Could you check a few things on this model? Use its own coordinates, in mm. A direction names the side the tool comes from. Round coordinates to 2 decimals unless told otherwise and drop trailing zeros. Loops run counter-clockwise (first coordinate to the right, second up) from the corner with the lowest first, then second, coordinate; pieces in that order, holes last. Notation, with made-up numbers: M -36,83.25 L -17,83.25 A9 cw -17,99.25 Z; hole C 77.5,-23.5 d11. An arc over 180 degrees is marked long. Answer in a Markdown table with one row per item.
```python
from build123d import *

# Parameters (mm, degrees)
SKETCH1_W           = 50
SKETCH1_H           = 170
BOSS_EXTRUDE1_DEPTH = 55
SKETCH2_W           = 34
SKETCH2_H           = 27
CUT_EXTRUDE1_DEPTH  = 181.416185527
SKETCH3_W           = 10
SKETCH3_H           = 24
SKETCH3_R           = 4.25
SKETCH3_R_2         = 1
CUT_EXTRUDE2_DEPTH  = 186.539753153
SKETCH4_W           = 2
SKETCH4_H           = 24
CUT_EXTRUDE3_DEPTH  = 178.623196683
SKETCH5_W           = 6.25
SKETCH5_H           = 11.25
CUT_EXTRUDE4_DEPTH  = 186.539753153
SKETCH6_W           = 38
SKETCH6_H           = 10
CUT_EXTRUDE5_DEPTH  = 181.416185527
SKETCH8_W           = 13.25
SKETCH8_H           = 2.25
CUT_EXTRUDE7_DEPTH  = 186.539753153
SKETCH9_W           = 34
SKETCH9_H           = 35.25
CUT_EXTRUDE8_DEPTH  = 179.297679458
SKETCH11_W          = 13.25
SKETCH11_H          = 20.25
CUT_EXTRUDE9_DEPTH  = 184.480414486
SKETCH12_W          = 28.5
SKETCH12_H          = 15
BOSS_EXTRUDE2_DEPTH = 8
SKETCH14_W          = 34
SKETCH14_H          = 15
SKETCH14_H_2        = 10.25
BOSS_EXTRUDE3_DEPTH = 13.25
SKETCH16_R          = 4.5
SKETCH16_R_2        = 2.5
CUT_EXTRUDE13_DEPTH = 8
SKETCH17_R          = 4.5
SKETCH17_W          = 55
SKETCH17_H          = 10.25
CUT_EXTRUDE15_DEPTH = 175.384811552
SKETCH18_W          = 71.25
SKETCH18_H          = 27.5
SKETCH18_W_2        = 13.75
SKETCH18_W_3        = 16.25
BOSS_EXTRUDE4_DEPTH = 50
SKETCH19_W          = 38
SKETCH19_H          = 7
CUT_EXTRUDE16_DEPTH = 152.25227271
SKETCH20_W          = 57.5
SKETCH20_H          = 27.5
CUT_EXTRUDE17_DEPTH = 102.137591923
CUT_EXTRUDE18_DEPTH = 100.39221549
SKETCH22_W          = 82.5
SKETCH22_H          = 2.5
BOSS_EXTRUDE5_DEPTH = 50
SKETCH24_W          = 22
SKETCH24_H          = 17
CUT_EXTRUDE19_DEPTH = 101.710289941
SKETCH25_W          = 38
SKETCH25_H          = 38.136363636
CUT_EXTRUDE20_DEPTH = 10


with BuildPart() as part:
    # Sketch1 → Boss-Extrude1 (new body)
    with BuildSketch(Plane.XY):
        with Locations((0, -85)):
            Rectangle(SKETCH1_W, SKETCH1_H)
    extrude(amount=-BOSS_EXTRUDE1_DEPTH)

    # Sketch2 → Cut-Extrude1 (cut, through all)
    with BuildSketch(Plane.XY):
        with Locations((0, -13.5)):
            Rectangle(SKETCH2_W, SKETCH2_H)
    extrude(amount=-CUT_EXTRUDE1_DEPTH, mode=Mode.SUBTRACT)

    # Sketch3 → Cut-Extrude2 (cut, through all)
    with BuildSketch(Plane(origin=(25, 0, 0), x_dir=(0, 0, -1), z_dir=(1, 0, 0))):
        with Locations((50, -12)):
            Rectangle(SKETCH3_W, SKETCH3_H)
        with Locations((5, -12)):
            Rectangle(SKETCH3_W, SKETCH3_H)
        with Locations(Location((27.5, -12.75, 0), (0, 0, 90))):
            Circle(SKETCH3_R)
        with Locations(Location((35.5, -12.75, 0), (0, 0, 90))):
            Circle(SKETCH3_R_2)
        with Locations(Location((27.5, -4.75, 0), (0, 0, 90))):
            Circle(SKETCH3_R_2)
        with Locations(Location((27.5, -20.75, 0), (0, 0, 90))):
            Circle(SKETCH3_R_2)
        with Locations(Location((19.5, -12.75, 0), (0, 0, 90))):
            Circle(SKETCH3_R_2)
    extrude(amount=-CUT_EXTRUDE2_DEPTH, mode=Mode.SUBTRACT)

    # Sketch4 → Cut-Extrude3 (cut, through all)
    with BuildSketch(Plane.XY.offset(-10)):
        with Locations((-18, -12)):
            Rectangle(SKETCH4_W, SKETCH4_H)
        with Locations((18, -12)):
            Rectangle(SKETCH4_W, SKETCH4_H)
    extrude(amount=-CUT_EXTRUDE3_DEPTH, mode=Mode.SUBTRACT)

    # Sketch5 → Cut-Extrude4 (cut, through all)
    with BuildSketch(Plane(origin=(25, 0, 0), x_dir=(0, 0, -1), z_dir=(1, 0, 0))):
        with BuildLine():
            Line((45, 0), (10, 0))
            Line((10, 0), (10, -12.75))
            Line((10, -12.75), (16.25, -12.75))
            ThreePointArc((16.25, -12.75), (27.5, -1.5), (38.75, -12.75))
            Line((38.75, -12.75), (45, -12.75))
            Line((45, -12.75), (45, 0))
        make_face()
        with Locations((13.125, -18.375)):
            Rectangle(SKETCH5_W, SKETCH5_H)
        with Locations((41.875, -18.375)):
            Rectangle(SKETCH5_W, SKETCH5_H)
    extrude(amount=-CUT_EXTRUDE4_DEPTH, mode=Mode.SUBTRACT)

    # Sketch6 → Cut-Extrude5 (cut, through all)
    with BuildSketch(Plane.XY):
        with Locations((0, -29)):
            Rectangle(SKETCH6_W, SKETCH6_H)
    extrude(amount=-CUT_EXTRUDE5_DEPTH, mode=Mode.SUBTRACT)

    # Sketch8 → Cut-Extrude7 (cut, through all)
    with BuildSketch(Plane(origin=(25, 0, 0), x_dir=(0, 0, -1), z_dir=(1, 0, 0))):
        with BuildLine():
            Line((27.5, -157.5), (27.5, -132.5))
            Line((27.5, -132.5), (13.25, -132.5))
            Line((13.25, -132.5), (13.25, -167.75))
            Line((13.25, -167.75), (17.25, -167.75))
            ThreePointArc((17.25, -167.75), (20.252155493, -160.502155493), (27.5, -157.5))
        make_face()
        with BuildLine():
            Line((41.75, -167.75), (41.75, -132.5))
            Line((41.75, -132.5), (27.5, -132.5))
            Line((27.5, -132.5), (27.5, -157.5))
            ThreePointArc((27.5, -157.5), (34.747844507, -160.502155493), (37.75, -167.75))
            Line((37.75, -167.75), (41.75, -167.75))
        make_face()
        with Locations((48.375, -168.875)):
            Rectangle(SKETCH8_W, SKETCH8_H)
        with Locations((6.625, -168.875)):
            Rectangle(SKETCH8_W, SKETCH8_H)
        with BuildLine():
            Line((17.25, -167.75), (13.25, -167.75))
            Line((13.25, -167.75), (13.25, -170))
            Line((13.25, -170), (17.5, -170))
            ThreePointArc((17.5, -170), (17.31269172, -168.881923142), (17.25, -167.75))
        make_face()
        with BuildLine():
            Line((41.75, -170), (41.75, -167.75))
            Line((41.75, -167.75), (37.75, -167.75))
            ThreePointArc((37.75, -167.75), (37.68730828, -168.881923142), (37.5, -170))
            Line((37.5, -170), (41.75, -170))
        make_face()
        with BuildLine():
            Line((27.5, -167.75), (27.5, -157.5))
            ThreePointArc((27.5, -157.5), (20.252155493, -160.502155493), (17.25, -167.75))
            Line((17.25, -167.75), (27.5, -167.75))
        make_face()
        with BuildLine():
            ThreePointArc((37.75, -167.75), (34.747844507, -160.502155493), (27.5, -157.5))
            Line((27.5, -157.5), (27.5, -167.75))
            Line((27.5, -167.75), (37.75, -167.75))
        make_face()
        with BuildLine():
            Line((27.5, -170), (27.5, -167.75))
            Line((27.5, -167.75), (17.25, -167.75))
            ThreePointArc((17.25, -167.75), (17.31269172, -168.881923142), (17.5, -170))
            Line((17.5, -170), (27.5, -170))
        make_face()
        with BuildLine():
            ThreePointArc((37.5, -170), (37.68730828, -168.881923142), (37.75, -167.75))
            Line((37.75, -167.75), (27.5, -167.75))
            Line((27.5, -167.75), (27.5, -170))
            Line((27.5, -170), (37.5, -170))
        make_face()
    extrude(amount=-CUT_EXTRUDE7_DEPTH, mode=Mode.SUBTRACT)

    # Sketch9 → Cut-Extrude8 (cut, through all)
    with BuildSketch(Plane.XY):
        with Locations((0, -150.125)):
            Rectangle(SKETCH9_W, SKETCH9_H)
    extrude(amount=-CUT_EXTRUDE8_DEPTH, mode=Mode.SUBTRACT)

    # Sketch11 → Cut-Extrude9 (cut, through all)
    with BuildSketch(Plane(origin=(25, 0, 0), x_dir=(0, 0, -1), z_dir=(1, 0, 0))):
        with BuildLine():
            ThreePointArc((17.25, -167.75), (20.252155493, -160.502155493), (27.5, -157.5))
            Line((27.5, -157.5), (27.5, -147.5))
            Line((27.5, -147.5), (13.25, -147.5))
            Line((13.25, -147.5), (13.25, -167.75))
            Line((13.25, -167.75), (17.25, -167.75))
        make_face()
        with BuildLine():
            Line((27.5, -147.5), (27.5, -157.5))
            ThreePointArc((27.5, -157.5), (34.747844507, -160.502155493), (37.75, -167.75))
            Line((37.75, -167.75), (41.75, -167.75))
            Line((41.75, -167.75), (41.75, -147.5))
            Line((41.75, -147.5), (27.5, -147.5))
        make_face()
        with Locations((48.375, -157.625)):
            Rectangle(SKETCH11_W, SKETCH11_H)
        with Locations((6.625, -157.625)):
            Rectangle(SKETCH11_W, SKETCH11_H)
    extrude(amount=-CUT_EXTRUDE9_DEPTH, mode=Mode.SUBTRACT)

    # Sketch12 → Boss-Extrude2 (add)
    with BuildSketch(Plane(origin=(25, 0, 0), x_dir=(0, 0, -1), z_dir=(1, 0, 0))):
        with Locations((27.5, -140)):
            Rectangle(SKETCH12_W, SKETCH12_H)
    boss_extrude2 = extrude(amount=-BOSS_EXTRUDE2_DEPTH)

    # Mirror1: Boss-Extrude2 across plane
    add(boss_extrude2.mirror(Plane(origin=(0, 0, 0), x_dir=(0, 0, 1), z_dir=(1, 0, 0))))

    # Sketch14 → Boss-Extrude3 (add)
    with BuildSketch(Plane.XY):
        with Locations((0, -140)):
            Rectangle(SKETCH14_W, SKETCH14_H)
        with Locations((0, -152.625)):
            Rectangle(SKETCH14_W, SKETCH14_H_2)
    boss_extrude3 = extrude(amount=-BOSS_EXTRUDE3_DEPTH)

    # Mirror2: Boss-Extrude3 across plane
    add(boss_extrude3.mirror(Plane.XY.offset(-27.5)))

    # Sketch16 → Cut-Extrude13 (cut)
    # profile 1 of 3: a face of its own
    with BuildSketch(Plane(origin=(25, 0, 0), x_dir=(0, 0, -1), z_dir=(1, 0, 0))):
        with Locations(Location((16.5, -135.75, 0), (0, 0, 90))):
            Circle(SKETCH16_R)
        with Locations((16.5, -135.75)):
            Circle(SKETCH16_R_2, mode=Mode.SUBTRACT)
    # profile 2 of 3: a face of its own
    with BuildSketch(Plane(origin=(25, 0, 0), x_dir=(0, 0, -1), z_dir=(1, 0, 0))):
        with Locations((16.5, -135.75)):
            Circle(SKETCH16_R_2)
    # profile 3 of 3: a face of its own
    with BuildSketch(Plane(origin=(25, 0, 0), x_dir=(0, 0, -1), z_dir=(1, 0, 0))):
        with Locations(Location((38.5, -135.75, 0), (0, 0, 90))):
            Circle(SKETCH16_R)
    cut_extrude13 = extrude(amount=-CUT_EXTRUDE13_DEPTH, mode=Mode.SUBTRACT)

    # Mirror3: Cut-Extrude13 across plane
    add(cut_extrude13.mirror(Plane(origin=(0, 0, 0), x_dir=(0, 0, 1), z_dir=(1, 0, 0))), mode=Mode.SUBTRACT)

    # Sketch17 → Cut-Extrude15 (cut, through all)
    # profile 1 of 4: a face of its own
    with BuildSketch(Plane(origin=(25, 0, 0), x_dir=(0, 0, -1), z_dir=(1, 0, 0))):
        Polygon((55, -51.5), (27.5, -51.5), (0, -51.5), (0, -147.5), (55, -147.5), align=None)
        with Locations((16.5, -135.75)):
            Circle(SKETCH17_R, mode=Mode.SUBTRACT)
        with Locations((38.5, -135.75)):
            Circle(SKETCH17_R, mode=Mode.SUBTRACT)
    # profile 2 of 4: a face of its own
    with BuildSketch(Plane(origin=(25, 0, 0), x_dir=(0, 0, -1), z_dir=(1, 0, 0))):
        with Locations((27.5, -152.625)):
            Rectangle(SKETCH17_W, SKETCH17_H)
    # profile 3 of 4: a face of its own
    with BuildSketch(Plane(origin=(25, 0, 0), x_dir=(0, 0, -1), z_dir=(1, 0, 0))):
        with Locations((38.5, -135.75)):
            Circle(SKETCH17_R)
    # profile 4 of 4: a face of its own
    with BuildSketch(Plane(origin=(25, 0, 0), x_dir=(0, 0, -1), z_dir=(1, 0, 0))):
        with Locations((16.5, -135.75)):
            Circle(SKETCH17_R)
    extrude(amount=-CUT_EXTRUDE15_DEPTH, mode=Mode.SUBTRACT)

    # Sketch18 → Boss-Extrude4 (add)
    with BuildSketch(Plane(origin=(25, 0, 0), x_dir=(0, 0, -1), z_dir=(1, 0, 0))):
        with Locations((-35.625, -37.75)):
            Rectangle(SKETCH18_W, SKETCH18_H)
        with Locations((61.875, -37.75)):
            Rectangle(SKETCH18_W_2, SKETCH18_H)
        Polygon((38.75, -51.5), (38.75, -24), (16.25, -24), (0, -24), (0, -51.5), align=None)
        with Locations((46.875, -37.75)):
            Rectangle(SKETCH18_W_3, SKETCH18_H)
    extrude(amount=-BOSS_EXTRUDE4_DEPTH)

    # Sketch19 → Cut-Extrude16 (cut, through all)
    with BuildSketch(Plane.XY.offset(71.25)):
        with Locations((0, -27.5)):
            Rectangle(SKETCH19_W, SKETCH19_H)
    extrude(amount=-CUT_EXTRUDE16_DEPTH, mode=Mode.SUBTRACT)

    # Sketch20 → Cut-Extrude17 (cut, through all)
    with BuildSketch(Plane(origin=(25, 0, 0), x_dir=(0, 0, -1), z_dir=(1, 0, 0))):
        with Locations((-42.5, -37.75)):
            Rectangle(SKETCH20_W, SKETCH20_H)
    extrude(amount=-CUT_EXTRUDE17_DEPTH, mode=Mode.SUBTRACT)

    # Sketch21 → Cut-Extrude18 (cut, through all)
    with BuildSketch(Plane(origin=(25, 0, 0), x_dir=(0, 0, -1), z_dir=(1, 0, 0))):
        Polygon((16.25, -24), (-13.75, -51.5), (-13.75, -24), align=None)
    extrude(amount=-CUT_EXTRUDE18_DEPTH, mode=Mode.SUBTRACT)

    # Sketch22 → Boss-Extrude5 (add)
    with BuildSketch(Plane(origin=(25, 0, 0), x_dir=(0, 0, -1), z_dir=(1, 0, 0))):
        with Locations((27.5, -52.75)):
            Rectangle(SKETCH22_W, SKETCH22_H)
    extrude(amount=-BOSS_EXTRUDE5_DEPTH)

    # Sketch24 → Cut-Extrude19 (cut, through all)
    with BuildSketch(Plane(origin=(25, 0, 0), x_dir=(0, 0, -1), z_dir=(1, 0, 0))):
        with Locations((57.75, -32.5)):
            Rectangle(SKETCH24_W, SKETCH24_H)
    extrude(amount=-CUT_EXTRUDE19_DEPTH, mode=Mode.SUBTRACT)

    # Sketch25 → Cut-Extrude20 (cut)
    with BuildSketch(Plane(origin=(0, -31, 0), x_dir=(1, 0, 0), z_dir=(0, 1, 0))):
        with Locations((0, 27.681818182)):
            Rectangle(SKETCH25_W, SKETCH25_H)
    extrude(amount=-CUT_EXTRUDE20_DEPTH, mode=Mode.SUBTRACT)


solid = part.part
```
1) If we mould it in two halves opening along X, with no side actions, what happens to faces 5 (the face through (-19, -26, -27)), 6 (the face through (25, -39, -27)), 7 (the face through (-22, -18, -16.25))? For each: released by +X, released by -X, zero draft, split by the parting line, or undercut.
Computed:
| item | result |
|---|---|
| face 5 | undercut |
| face 6 | released by +X |
| face 7 | zero draft |
2) I need wall thicknesses on line 1 (Z direction, x = -21.7, y = -12.75); line 2 (X direction, y = -28, z = -12.5); line 3 (Y direction, x = -4, z = -33). Which ranges of each line are inside material? Lowest first, please.
Computed:
| item | result |
|---|---|
| line 1 | z = -38.75 to -36.5, -34.5 to -31.75, -23.25 to -20.5, -18.5 to -16.25 |
| line 2 | x = -25 to -19, 19 to 25 |
| line 3 | y = -54 to -41 |
3) I want a section at C-C, the plane z = -27.5. State how many separate pieces and enclosed holes the cut face has, plus the area to 3 significant figures.
Computed:
| item | result |
|---|---|
| separate pieces | 7 |
| enclosed holes | 0 |
| area | 974 mm² |
4) I want a section at A-A, the plane y = -20.75. Please give me the cut outline in (x, z), plus the area to 3 significant figures.
Computed:
| item | result |
|---|---|
| outline | M -25,-38.75 L -19,-38.75 L -19,-28.5 L -25,-28.5 Z; M -25,-26.5 L -19,-26.5 L -19,-16.25 L -25,-16.25 Z; M 19,-38.75 L 25,-38.75 L 25,-28.5 L 19,-28.5 Z; M 19,-26.5 L 25,-26.5 L 25,-16.25 L 19,-16.25 Z |
| area | 246 mm² |
5) I want a section at D-D, the plane y = -28. Please give me the cut outline in (x, z), plus the area to 3 significant figures.
Computed:
| item | result |
|---|---|
| outline | M -25,-46.75 L -19,-46.75 L -19,-11.89 L -25,-11.89 Z; M 19,-46.75 L 25,-46.75 L 25,-11.89 L 19,-11.89 Z |
| area | 418 mm² |
6) I want a section at B-B, the plane z = -41. Please give me the cut outline in (x, y), plus the area to 3 significant figures.
Computed:
| item | result |
|---|---|
| outline | M -25,-54 L 25,-54 L 25,-24 L 19,-24 L 19,-41 L -19,-41 L -19,-24 L -25,-24 Z |
| area | 854 mm² |
7) Which directions (+Z, -Z, +X, -X, +Y, -Y) give clear straight access to the entire face, cutting with the end or side of a thin tool? Please do faces 1 (the face through (22, -18, -38.75)), 2 (the face through (22, -18, -16.25)), 3 (the face through (0, -36, -8.614)), 4 (the face through (22.04, -4.88, -26.51)).
Computed:
| item | result |
|---|---|
| face 1 | -Z, +X, -X, +Y |
| face 2 | +Z, +X, -X, +Y |
| face 3 | -Z, +Y |
| face 4 | +X, -X |
8) Will these pins go through, and if not, where does the flat tip stop? P1, Ø6.5, axis at x = -22, y = -31, coming from the -Z side; P2, Ø6.5, axis at x = -21.5, z = -41, coming from the +Y side; P3, Ø1, axis at x = 6, z = -33.5, coming from the +Y side.
Computed:
| item | result |
|---|---|
| P1 | stops at z = -46.75 |
| P2 | stops at y = -8.11 |
| P3 | stops at y = -41 |
